```python
from build123d import *

# Parameters (mm, degrees)
F1_DEPTH      = 19.05
F0_R          = 1.9939
F2_DEPTH      = 2.54
F3_W          = 2.54
F3_H          = 1.905
F4_DEPTH      = 8.89
F5_W          = 2.54
F5_H          = 1.905
F6_DEPTH      = 11.43
F7_W          = 2.54
F7_H          = 2.54
F8_W          = 2.54
F8_H          = 2.54
F9_DEPTH      = 10.16
F10_W         = 2.54
F10_H         = 2.54
F11_DEPTH     = 11.43
F12_T1_DEPTH  = 9.525
F12_T3_DEPTH  = 14.605
F12_T5_DEPTH  = 26.035
F12_T7_DEPTH  = 9.525
F12_T9_DEPTH  = 4.445
F12_T11_DEPTH = 19.685
F12_T13_DEPTH = 22.225
F12_T15_DEPTH = 8.89
F12_T17_DEPTH = 8.89
F12_T19_DEPTH = 8.89
F12_S23_W     = 1.27
F12_S23_H     = 1.27
F12_T24_DEPTH = 1.27
F12_S29_W     = 1.27
F12_S29_H     = 1.27
F12_T30_DEPTH = 1.27


# Not quite as in the source:
# - a fillet or chamfer that OpenCascade refuses, or shapes differently, is made with other operations: its cross-section is extruded or revolved along the edge and cut away or added


with BuildPart() as f1:
    # F0 (on Front) → F1 (new body)
    with BuildSketch(Plane.XZ):
        Polygon((-23.2056408978, -6.35), (-23.2056408978, 0), (-25.7456408978, 0), (-25.7456408978, -8.89), (-9.8706408978, -8.89), (-9.8706408978, 0), (-12.4106408978, 0), (-12.4106408978, -6.35), align=None)
    extrude(amount=F1_DEPTH)

    # F0 (on Front) → F2 (join)
    with BuildSketch(Plane.XZ):
        Polygon((-25.7456408978, -8.89), (-25.7456408978, 0), (-32.0956408978, 0), (-32.0956408978, -12.7), (-3.5206408978, -12.7), (-3.5206408978, 0), (-9.8706408978, 0), (-9.8706408978, -8.89), align=None)
        with Locations((-28.2856408978, -3.81)):
            Circle(F0_R, mode=Mode.SUBTRACT)
        with Locations((-7.3306408978, -3.81)):
            Circle(F0_R, mode=Mode.SUBTRACT)
    extrude(amount=F2_DEPTH)

    # F3 (on face) → F4 (join)
    with BuildSketch(Plane.XZ.offset(19.05)):
        with Locations((-11.1406408978, -3.4925)):
            Rectangle(F3_W, F3_H)
        with Locations((-24.4756408978, -3.4925)):
            Rectangle(F3_W, F3_H)
    extrude(amount=F4_DEPTH)

    # F5 (on face) → F6 (join)
    with BuildSketch(Plane(origin=(-12.4106408978, 0, 0), x_dir=(0, -1, 0), z_dir=(-1, 0, 0))):
        with Locations((26.67, -3.4925)):
            Rectangle(F5_W, F5_H)
    extrude(amount=F6_DEPTH)

    # F7 (on face) + F8 (on face) → F9 (join)
    with BuildSketch(Plane.XY):
        with Locations((-24.4756408978, -11.43)):
            Rectangle(F7_W, F7_H)
    with BuildSketch(Plane.XY):
        with Locations((-11.1406408978, -11.43)):
            Rectangle(F8_W, F8_H)
    extrude(amount=F9_DEPTH)

    # F10 (on face) → F11 (join)
    with BuildSketch(Plane.YZ.offset(-23.2056408978)):
        with Locations((-11.43, 8.89)):
            Rectangle(F10_W, F10_H)
    extrude(amount=F11_DEPTH)

    # F12: fillet of radius 1.27 on 18 edges, made by hand

    # F12_s2 → F12_t1 (cut)
    with BuildSketch(Plane.YZ.offset(-35.2706408978)):
        with BuildLine():
            ThreePointArc((-1.27, 0), (-2.1680256121, -0.3719743879), (-2.54, -1.27))
            Line((-2.54, -1.27), (-2.54, 0))
            Line((-2.54, 0), (-1.27, 0))
        make_face()
    extrude(amount=F12_T1_DEPTH, mode=Mode.SUBTRACT)

    # F12_s4 → F12_t3 (cut)
    with BuildSketch(Plane.XY.offset(-11.43)):
        with BuildLine():
            ThreePointArc((-32.0956408978, -1.27), (-31.7236665099, -2.1680256121), (-30.8256408978, -2.54))
            Line((-30.8256408978, -2.54), (-32.0956408978, -2.54))
            Line((-32.0956408978, -2.54), (-32.0956408978, -1.27))
        make_face()
        with BuildLine():
            ThreePointArc((-3.5206408978, -1.27), (-3.8926152856, -2.1680256121), (-4.7906408978, -2.54))
            Line((-4.7906408978, -2.54), (-3.5206408978, -2.54))
            Line((-3.5206408978, -2.54), (-3.5206408978, -1.27))
        make_face()
    extrude(amount=F12_T3_DEPTH, mode=Mode.SUBTRACT)

    # F12_s6 → F12_t5 (cut)
    with BuildSketch(Plane.YZ.offset(-30.8256408978)):
        with BuildLine():
            ThreePointArc((-1.27, -12.7), (-2.1680256121, -12.3280256121), (-2.54, -11.43))
            Line((-2.54, -11.43), (-2.54, -12.7))
            Line((-2.54, -12.7), (-1.27, -12.7))
        make_face()
    extrude(amount=F12_T5_DEPTH, mode=Mode.SUBTRACT)

    # F12_s8 → F12_t7 (cut)
    with BuildSketch(Plane.YZ.offset(-9.8706408978)):
        with BuildLine():
            ThreePointArc((-1.27, 0), (-2.1680256121, -0.3719743879), (-2.54, -1.27))
            Line((-2.54, -1.27), (-2.54, 0))
            Line((-2.54, 0), (-1.27, 0))
        make_face()
    extrude(amount=F12_T7_DEPTH, mode=Mode.SUBTRACT)

    # F12_s10 → F12_t9 (cut)
    with BuildSketch(Plane.XZ.offset(-3.175)):
        with BuildLine():
            ThreePointArc((-4.7906408978, -12.7), (-3.8926152856, -12.3280256121), (-3.5206408978, -11.43))
            Line((-3.5206408978, -11.43), (-3.5206408978, -12.7))
            Line((-3.5206408978, -12.7), (-4.7906408978, -12.7))
        make_face()
        with BuildLine():
            ThreePointArc((-32.0956408978, -11.43), (-31.7236665099, -12.3280256121), (-30.8256408978, -12.7))
            Line((-30.8256408978, -12.7), (-32.0956408978, -12.7))
            Line((-32.0956408978, -12.7), (-32.0956408978, -11.43))
        make_face()
    extrude(amount=F12_T9_DEPTH, mode=Mode.SUBTRACT)

    # F12_s12 → F12_t11 (cut)
    with BuildSketch(Plane.XZ.offset(2.54)):
        with BuildLine():
            ThreePointArc((-9.8706408978, -7.62), (-10.2426152856, -8.5180256121), (-11.1406408978, -8.89))
            Line((-11.1406408978, -8.89), (-9.8706408978, -8.89))
            Line((-9.8706408978, -8.89), (-9.8706408978, -7.62))
        make_face()
        with BuildLine():
            ThreePointArc((-25.7456408978, -7.62), (-25.3736665099, -8.5180256121), (-24.4756408978, -8.89))
            Line((-24.4756408978, -8.89), (-25.7456408978, -8.89))
            Line((-25.7456408978, -8.89), (-25.7456408978, -7.62))
        make_face()
    extrude(amount=F12_T11_DEPTH, mode=Mode.SUBTRACT)

    # F12_s14 → F12_t13 (cut)
    with BuildSketch(Plane.YZ.offset(-28.9206408978)):
        with BuildLine():
            ThreePointArc((-26.67, -2.54), (-27.5680256121, -2.9119743879), (-27.94, -3.81))
            Line((-27.94, -3.81), (-27.94, -2.54))
            Line((-27.94, -2.54), (-26.67, -2.54))
        make_face()
        with BuildLine():
            ThreePointArc((-19.05, -7.62), (-18.6780256121, -8.5180256121), (-17.78, -8.89))
            Line((-17.78, -8.89), (-19.05, -8.89))
            Line((-19.05, -8.89), (-19.05, -7.62))
        make_face()
        with BuildLine():
            ThreePointArc((-27.94, -3.175), (-27.5680256121, -4.0730256121), (-26.67, -4.445))
            Line((-26.67, -4.445), (-27.94, -4.445))
            Line((-27.94, -4.445), (-27.94, -3.175))
        make_face()
        with BuildLine():
            ThreePointArc((-11.43, 10.16), (-12.3280256121, 9.7880256121), (-12.7, 8.89))
            Line((-12.7, 8.89), (-12.7, 10.16))
            Line((-12.7, 10.16), (-11.43, 10.16))
        make_face()
        with BuildLine():
            ThreePointArc((-10.16, 8.89), (-10.5319743879, 9.7880256121), (-11.43, 10.16))
            Line((-11.43, 10.16), (-10.16, 10.16))
            Line((-10.16, 10.16), (-10.16, 8.89))
        make_face()
    extrude(amount=F12_T13_DEPTH, mode=Mode.SUBTRACT)

    # F12_s16 → F12_t15 (cut)
    with BuildSketch(Plane.YZ.offset(-28.9206408978)):
        with BuildLine():
            ThreePointArc((-19.05, -1.27), (-18.6780256121, -0.3719743879), (-17.78, 0))
            Line((-17.78, 0), (-19.05, 0))
            Line((-19.05, 0), (-19.05, -1.27))
        make_face()
    extrude(amount=F12_T15_DEPTH, mode=Mode.SUBTRACT)

    # F12_s18 → F12_t17 (cut)
    with BuildSketch(Plane.YZ.offset(-15.5856408978)):
        with BuildLine():
            ThreePointArc((-17.78, 0), (-18.6780256121, -0.3719743879), (-19.05, -1.27))
            Line((-19.05, -1.27), (-19.05, 0))
            Line((-19.05, 0), (-17.78, 0))
        make_face()
    extrude(amount=F12_T17_DEPTH, mode=Mode.SUBTRACT)

    # F12_s20 → F12_t19 (cut)
    with BuildSketch(Plane.XZ.offset(6.985)):
        with BuildLine():
            ThreePointArc((-25.7456408978, 8.89), (-25.3736665099, 9.7880256121), (-24.4756408978, 10.16))
            Line((-24.4756408978, 10.16), (-25.7456408978, 10.16))
            Line((-25.7456408978, 10.16), (-25.7456408978, 8.89))
        make_face()
        with BuildLine():
            ThreePointArc((-9.8706408978, 8.89), (-10.2426152856, 9.7880256121), (-11.1406408978, 10.16))
            Line((-11.1406408978, 10.16), (-9.8706408978, 10.16))
            Line((-9.8706408978, 10.16), (-9.8706408978, 8.89))
        make_face()
    extrude(amount=F12_T19_DEPTH, mode=Mode.SUBTRACT)


with BuildPart() as f12_tool22:
    # F12_s23 → F12_t24 (new body)
    with BuildSketch(Plane.YZ.offset(-30.8256408978)):
        with Locations((-1.905, -12.065)):
            Rectangle(F12_S23_W, F12_S23_H)
    extrude(amount=-F12_T24_DEPTH)

    # F12_s25 → F12_t26 (revolve, cut)
    with BuildSketch(Plane(origin=(-30.8256408978, -1.27, -11.43), x_dir=(0, 0.7071067812, 0.7071067812), z_dir=(0, -0.7071067812, 0.7071067812))):
        with BuildLine():
            ThreePointArc((0, -1.27), (1.27, 0), (0, 1.27))
            Line((0, 1.27), (0, -1.27))
        make_face()
    revolve(axis=Axis((-30.8256408978, -1.27, -11.43), (-1, 0, 0)), mode=Mode.SUBTRACT)


with BuildPart() as f1_1:
    add(f1.part)

    # F12_t21: cut F12_tool22
    add(f12_tool22.part, mode=Mode.SUBTRACT)


with BuildPart() as f12_tool28:
    # F12_s29 → F12_t30 (new body)
    with BuildSketch(Plane.YZ.offset(-4.7906408978)):
        with Locations((-1.905, -12.065)):
            Rectangle(F12_S29_W, F12_S29_H)
    extrude(amount=F12_T30_DEPTH)

    # F12_s31 → F12_t32 (revolve, cut)
    with BuildSketch(Plane(origin=(-4.7906408978, -1.27, -11.43), x_dir=(0, 0.7071067812, 0.7071067812), z_dir=(0, 0.7071067812, -0.7071067812))):
        with BuildLine():
            ThreePointArc((0, -1.27), (1.27, 0), (0, 1.27))
            Line((0, 1.27), (0, -1.27))
        make_face()
    revolve(axis=Axis((-4.7906408978, -1.27, -11.43), (1, 0, 0)), mode=Mode.SUBTRACT)


with BuildPart() as f1_2:
    add(f1_1.part)

    # F12_t27: cut F12_tool28
    add(f12_tool28.part, mode=Mode.SUBTRACT)


solid = f1_2.part
```
Model file for the job. Use its own axes, mm. A direction names the side the tool comes from. Coordinates: 2 decimals unless noted, no trailing zeros. Loops run counter-clockwise (first coordinate to the right, second up) from the corner with the lowest first, then second, coordinate; pieces in that order, holes last. Notation, with made-up numbers: M 13,-5.75 L 55,-5.75 A27 ccw 55,20.25 Z; hole C -0.5,-37.5 d4. An arc over 180 degrees is marked long. Use CSV: the item, a comma, the result in double quotes. Start each with the question number.
1. Band-saw the part on C-C, the plane y = -25. List the corners of the cut face in (x, z) (3 decimals), then the cut area to 3 significant figures.
2. Probe probe 1 along Y at (x, z) = (-28.75, -11.5); probe 2 along Y at (x, z) = (-25.25, -5.5); probe 3 along Z at (x, y) = (-18.25, -1.25). List the from-to ranges inside material, lowest first. Write a range as [from, to].
3. Flat gauge pins, fed straight in: pin 1 (1.3 mm diameter, centred on x = -11.5, y = -15, fed in from +Z); pin 2 (10 mm diameter, centred on x = -15, z = 3, fed in from -Y); pin 3 (4 mm diameter, centred on y = -4, z = -3, fed in from +X). Where does each tip first touch, or does it go through?
4. Two-plate mould, pull along Z, no slides. Class faces 1 (the flat face through (-18, -11, 7.62)), 2 (the flat face through (-18, -10, -8.89)), 3 (the flat face through (-11, -15, 0)): pulls with the +Z half, pulls with the -Z half, needs draft (parallel to the pull), parting line crosses it, or undercut.
5. Band-saw the part on D-D, the plane x = -29.75. List the corners of the cut face in (y, z).
6. Tool access for faces 4 (the flat face through (-18, -2.54, -10)), 5 (the flat face through (-11, -19.05, -2)), 6 (the flat face through (-16, -26, -4.445)): list every direction of +Z, -Z, +X, -X, +Y, -Y with a clear straight run to the whole face (end or side of a thin tool).
7. Band-saw the part on A-A, the plane z = 1.5. List the corners of the cut face in (x, y), then the cut area to 3 significant figures.
8. Band-saw the part on B-B, the plane x = -21.75. Give the number of separate pieces and of enclosed holes in the cut face, then the cut area to 3 significant figures.
Entries:
1,outline,"M -25.746,-4.445 L -23.206,-4.445 L -23.206,-2.54 L -25.746,-2.54 Z; M -12.411,-4.445 L -9.871,-4.445 L -9.871,-2.54 L -12.411,-2.54 Z"
1,area,"9.68 mm2"
2,probe 1,"y = [-2.54, 0]"
2,probe 2,"y = [-19.05, 0]"
2,probe 3,"z = [-12.7, -6.35]"
3,pin 1,"stops at z = 0"
3,pin 2,"stops at y = -19.05"
3,pin 3,"stops at x = -3.75"
4,face 1,"undercut"
4,face 2,"pulls with the -Z half"
4,face 3,"pulls with the +Z half"
5,outline,"M -2.54,-11.43 A1.27 ccw -1.27,-12.7 L 0,-12.7 L 0,-5.16 L -2.54,-5.16 Z; M -2.54,-2.46 L 0,-2.46 L 0,0 L -1.27,0 A1.27 ccw -2.54,-1.27 Z"
6,face 4,"-Z, -Y"
6,face 5,"+Z, +X, -X, -Y"
6,face 6,"-Z, +X, -X, -Y"
7,outline,"M -25.75,-12.7 L -23.21,-12.7 L -23.21,-10.16 L -25.75,-10.16 Z; M -12.41,-12.7 L -9.87,-12.7 L -9.87,-10.16 L -12.41,-10.16 Z"
7,area,"12.9 mm2"
8,separate pieces,"3"
8,enclosed holes,"0"
8,area,"67.3 mm2"
